The figure shows three views and two pictorial views of one solid part (mm, origin at its lowest corner). Answer the questions. Give positions to 0.01 mm unless a question says otherwise; leave off trailing zeros. Loops run counter-clockwise (first coordinate to the right, second up) from the corner with the lowest first, then second, coordinate; pieces in that order, holes last. Notation, with made-up numbers: (87.5, 78.25) - (112.5, 78.25) arc R18 cw to (112.5, 82.25) - close; hole circle Ø6 at (-2, 42). An arc over 180 degrees is marked (long way). Write each question's results on one line, items separated by ' | '.
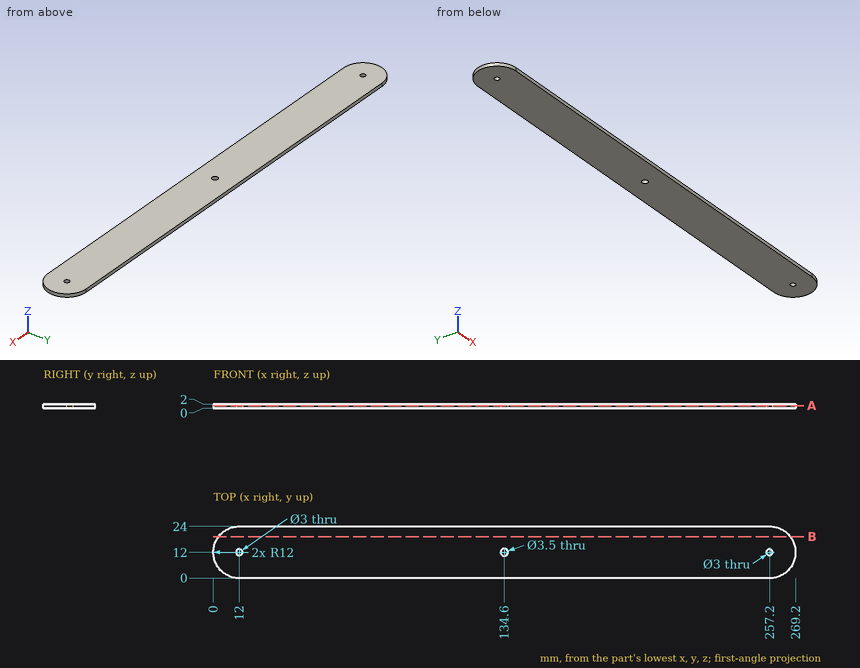
Item 1: A cutting plane is placed at B-B, the plane y = 19.25. Determine the outline of the cut face in (x, z), plus the area to 3 significant figures.
Values found:
outline: (2.44, 0) - (266.76, 0) - (266.76, 2) - (2.44, 2) - close | area: 529 mm²
Item 2: Find the intervals of material crossed by line 1 along Y through (x, z) = (257.2, 1.45); line 2 along Y through (x, z) = (134.6, 0.7); line 3 along X through (y, z) = (12.75, 0.75), in increasing order. Write a range as [from, to].
Values found:
line 1: y = [0, 10.5], [13.5, 24] | line 2: y = [0, 10.25], [13.75, 24] | line 3: x = [0.02, 10.7], [13.3, 133.02], [136.18, 255.9], [258.5, 269.18]
Item 3: A cutting plane is placed at A-A, the plane z = 1.25. Determine the outline of the cut face in (x, y).
Values found:
outline: (12, 0) - (257.2, 0) arc R12 ccw to (257.2, 24) - (12, 24) arc R12 ccw to start; hole circle Ø3 at (12, 12); hole circle Ø3.5 at (134.6, 12); hole circle Ø3 at (257.2, 12)
Item 4: A flat-ended cylindrical pin translates along its axis: P1, Ø2, axis at x = 134.6, y = 12, coming from the -Z side. Find the tip coordinate at first contact, or state that the pin passes through.
Values found:
P1: passes through
